Autodesk Inventor part; units mm, degrees
ref_plane "YZ Plane" through (0, 0, 0) normal (1, 0, 0) x (0, 1, 0)
ref_plane "XZ Plane" through (0, 0, 0) normal (0, 1, 0) x (-1, 0, 0)
ref_plane "XY Plane" through (0, 0, 0) normal (0, 0, 1) x (1, 0, 0)
sketch "Sketch1" plane through (0, 0, 0) normal (0, 0, 1) x (1, 0, 0)
  line L0 (6, 6) -> (200, 6)
  line L1 (200, 6) -> (200, 200)
  line L2 (200, 200) -> (42, 200)
  line L3 (6, 83) -> (6, 6)
  line L4 (6, 6) -> (56, 6)
  line L5 (200, 6) -> (150, 6)
  line L6 (200, 6) -> (200, 153)
  line L7 (150, 6) -> (142.5, 6)
  line L8 (200, 6) -> (200, 166)
  arc A0 (152.5, 174.3333) -> (147.5, 174.3333) centre (150, 174.3333) ccw
  line L9 (150, 6) -> (50, 6)
  arc A1 (47.8689, 14.6053) -> (52.8158, 14.5813) centre (50.3406, 14.23) ccw
  arc A2 (53.8259, 22.009) -> (52.8051, 13.8106) centre (86.918, 13.7258) ccw
  arc A3 (51.3944, 191.2047) -> (46.3962, 191.0801) centre (48.8946, 191.1682) ccw
  line L10 (53.8599, 22.4199) -> (51.3944, 191.2047)
  line L11 (48.8556, 22.7156) -> (46.3962, 191.0801)
  arc A4 (53.7373, 21.6465) -> (53.8589, 22.4929) centre (51.3599, 22.4199) ccw
  arc A5 (48.8556, 22.7156) -> (47.8689, 14.6053) centre (80.6169, 14.7362) ccw
  line L12 (52.8406, 14.23) -> (52.8088, 14.23)
  arc A6 (147.5, 14.23) -> (152.5, 14.23) centre (150, 14.23) ccw
  line L13 (147.5, 14.23) -> (147.5, 174.3333)
  line L14 (152.5, 14.23) -> (152.5, 174.3333)
  line L15 (42, 83) -> (6, 83)
  line L16 (42, 200) -> (39, 200)
  line L17 (39, 200) -> (39, 180)
  line L18 (39, 160) -> (39, 140)
  line L19 (39, 120) -> (39, 100)
  line L20 (39, 100) -> (42, 100)
  line L21 (39, 120) -> (42, 120)
  line L22 (39, 140) -> (42, 140)
  line L23 (39, 160) -> (42, 160)
  line L24 (39, 180) -> (42, 180)
  line L25 (39, 120) -> (39, 100)
  line L26 (39, 200) -> (39, 180)
  line L27 (39, 160) -> (39, 140)
  line L28 (42, 180) -> (42, 160)
  line L29 (42, 140) -> (42, 120)
  line L30 (42, 100) -> (42, 83)
  dimension "d1" = 194
extrude "Extrusion1" add sketch "Sketch1" along normal blind 3
sketch "Sketch2" plane through (0, 0, 3) normal (0, 0, 1) x (1, 0, 0)
  line L0 (200, 6) -> (200, 200)
  line L1 (200, 200) -> (39, 200)
  line L2 (42, 180) -> (42, 160)
  line L3 (42, 83) -> (6, 83)
  line L4 (6, 83) -> (6, 6)
  line L5 (6, 6) -> (200, 6)
  line L6 (147.5, 14.23) -> (147.5, 174.3333)
  arc A0 (152.5, 174.3333) -> (147.5, 174.3333) centre (150, 174.3333) ccw
  line L7 (152.5, 174.3333) -> (152.5, 14.23)
  arc A1 (147.5, 14.23) -> (152.5, 14.23) centre (150, 14.23) ccw
  arc A2 (51.3944, 191.2047) -> (46.3962, 191.0801) centre (48.8946, 191.1682) ccw
  line L8 (51.3944, 191.2047) -> (53.8589, 22.4929)
  arc A3 (53.7373, 21.6465) -> (53.8589, 22.4929) centre (51.3599, 22.4199) ccw
  arc A4 (53.7373, 21.6465) -> (52.8158, 14.5813) centre (86.918, 13.7258) ccw
  arc A5 (47.8689, 14.6053) -> (52.8158, 14.5813) centre (50.3406, 14.23) ccw
  arc A6 (48.8556, 22.7156) -> (47.8689, 14.6053) centre (80.6169, 14.7362) ccw
  line L9 (48.8556, 22.7156) -> (46.3962, 191.0801)
  line L10 (6, 6) -> (33, 6)
  line L11 (33, 6) -> (53, 6)
  line L12 (53, 6) -> (73, 6)
  line L13 (73, 6) -> (93, 6)
  line L14 (93, 6) -> (113, 6)
  line L15 (113, 6) -> (133, 6)
  line L16 (133, 6) -> (153, 6)
  line L17 (153, 6) -> (173, 6)
  line L18 (6, 6) -> (6, 9)
  line L19 (33, 6) -> (33, 3)
  line L20 (173, 6) -> (173, 3)
  line L21 (53, 6) -> (53, 3)
  line L22 (93, 6) -> (93, 3)
  line L23 (73, 6) -> (73, 3)
  line L24 (133, 6) -> (133, 3)
  line L25 (113, 6) -> (113, 3)
  line L26 (153, 6) -> (153, 3)
  line L27 (6, 6) -> (6, 3)
  line L28 (6, 3) -> (33, 3)
  line L29 (173, 3) -> (200, 3)
  line L30 (200, 3) -> (200, 6.6126)
  line L31 (73, 3) -> (53, 3)
  line L32 (153, 3) -> (133, 3)
  line L33 (113, 3) -> (93, 3)
  line L34 (39, 200) -> (39, 180)
  line L35 (39, 180) -> (42, 180)
  line L36 (42, 160) -> (39, 160)
  line L37 (39, 160) -> (39, 140)
  line L38 (39, 140) -> (42, 140)
  line L39 (42, 140) -> (42, 120)
  line L40 (42, 120) -> (39, 120)
  line L41 (39, 120) -> (39, 100)
  line L42 (39, 100) -> (42, 100)
  line L43 (42, 100) -> (42, 83)
  point P0 (120.702, 9)
  point P1 (49.056, 9)
extrude "Extrusion2" add sketch "Sketch2" against normal blind 3 contours L30 L29 L20 L5 | L26 L32 L24 L5 | L25 L33 L22 L5 | L23 L31 L21 L5 | L19 L28 L27 L5
sketch "Sketch3" plane through (0, 0, 3) normal (0, 0, 1) x (1, 0, 0)
  line L0 (153, 6) -> (173, 6)
  line L1 (113, 6) -> (133, 6)
  line L2 (200, 3) -> (200, 200)
  line L3 (200, 200) -> (39, 200)
  line L4 (42, 180) -> (42, 160)
  line L5 (42, 83) -> (6, 83)
  line L6 (6, 83) -> (6, 3)
  line L7 (73, 6) -> (93, 6)
  line L8 (33, 6) -> (53, 6)
  line L9 (147.5, 14.23) -> (147.5, 174.3333)
  arc A0 (152.5, 174.3333) -> (147.5, 174.3333) centre (150, 174.3333) ccw
  line L10 (152.5, 174.3333) -> (152.5, 14.23)
  arc A1 (147.5, 14.23) -> (152.5, 14.23) centre (150, 14.23) ccw
  arc A2 (51.3944, 191.2047) -> (46.3962, 191.0801) centre (48.8946, 191.1682) ccw
  line L11 (51.3944, 191.2047) -> (53.8589, 22.4929)
  arc A3 (53.7373, 21.6465) -> (53.8589, 22.4929) centre (51.3599, 22.4199) ccw
  arc A4 (53.7373, 21.6465) -> (52.8158, 14.5813) centre (86.918, 13.7258) ccw
  arc A5 (47.8689, 14.6053) -> (52.8158, 14.5813) centre (50.3406, 14.23) ccw
  arc A6 (48.8556, 22.7156) -> (47.8689, 14.6053) centre (80.6169, 14.7362) ccw
  line L12 (48.8556, 22.7156) -> (46.3962, 191.0801)
  line L13 (6, 83) -> (6, 80)
  line L14 (6, 83) -> (3, 83)
  line L15 (3, 6) -> (3, 14.5)
  line L16 (3, 83) -> (3, 74.5)
  line L17 (3, 54.5) -> (3, 34.5)
  line L18 (3, 74.5) -> (6, 74.5)
  line L19 (3, 54.5) -> (6, 54.5)
  line L20 (3, 34.5) -> (6, 34.5)
  line L21 (3, 14.5) -> (6, 14.5)
  line L22 (3, 14.5) -> (3, 6)
  line L23 (3, 83) -> (3, 74.5)
  line L24 (3, 54.5) -> (3, 34.5)
  line L25 (3, 6) -> (3, 3)
  line L26 (3, 3) -> (6, 3)
  line L27 (6, 3) -> (6, 6)
  line L28 (6, 3) -> (33, 3)
  line L29 (33, 3) -> (33, 6)
  line L30 (53, 6) -> (53, 3)
  line L31 (53, 3) -> (73, 3)
  line L32 (73, 3) -> (73, 6)
  line L33 (93, 6) -> (93, 3)
  line L34 (93, 3) -> (113, 3)
  line L35 (113, 3) -> (113, 6)
  line L36 (133, 6) -> (133, 3)
  line L37 (133, 3) -> (153, 3)
  line L38 (153, 3) -> (153, 6)
  line L39 (173, 6) -> (173, 3)
  line L40 (173, 3) -> (200, 3)
  line L41 (39, 200) -> (39, 180)
  line L42 (39, 180) -> (42, 180)
  line L43 (42, 160) -> (39, 160)
  line L44 (39, 160) -> (39, 140)
  line L45 (39, 140) -> (42, 140)
  line L46 (42, 140) -> (42, 120)
  line L47 (42, 120) -> (39, 120)
  line L48 (39, 120) -> (39, 100)
  line L49 (39, 100) -> (42, 100)
  line L50 (42, 100) -> (42, 83)
  point P0 (6, 3)
  dimension "d43" = 3
extrude "Extrusion3" add sketch "Sketch3" against normal blind 3 contours L26 L25 L15 L21 L6 | L6 L18 L16 L14 | L20 L17 L19 L6
sketch "Sketch4" plane through (0, 0, 3) normal (0, 0, 1) x (1, 0, 0)
  line L0 (153, 6) -> (173, 6)
  line L1 (113, 6) -> (133, 6)
  line L2 (200, 200) -> (39, 200)
  line L3 (42, 180) -> (42, 160)
  line L4 (42, 83) -> (3, 83)
  line L5 (3, 83) -> (3, 74.5)
  line L6 (3, 74.5) -> (6, 74.5)
  line L7 (6, 74.5) -> (6, 54.5)
  line L8 (6, 54.5) -> (3, 54.5)
  line L9 (3, 54.5) -> (3, 34.5)
  line L10 (3, 34.5) -> (6, 34.5)
  line L11 (73, 6) -> (93, 6)
  line L12 (33, 6) -> (53, 6)
  line L13 (147.5, 14.23) -> (147.5, 174.3333)
  arc A0 (152.5, 174.3333) -> (147.5, 174.3333) centre (150, 174.3333) ccw
  line L14 (152.5, 174.3333) -> (152.5, 14.23)
  arc A1 (147.5, 14.23) -> (152.5, 14.23) centre (150, 14.23) ccw
  arc A2 (51.3944, 191.2047) -> (46.3962, 191.0801) centre (48.8946, 191.1682) ccw
  line L15 (51.3944, 191.2047) -> (53.8589, 22.4929)
  arc A3 (53.7373, 21.6465) -> (53.8589, 22.4929) centre (51.3599, 22.4199) ccw
  arc A4 (53.7373, 21.6465) -> (52.8158, 14.5813) centre (86.918, 13.7258) ccw
  arc A5 (47.8689, 14.6053) -> (52.8158, 14.5813) centre (50.3406, 14.23) ccw
  arc A6 (48.8556, 22.7156) -> (47.8689, 14.6053) centre (80.6169, 14.7362) ccw
  line L16 (48.8556, 22.7156) -> (46.3962, 191.0801)
  line L17 (200, 200) -> (203, 200)
  line L18 (200, 6) -> (200, 33)
  line L19 (200, 33) -> (200, 53)
  line L20 (200, 53) -> (200, 73)
  line L21 (200, 73) -> (200, 93)
  line L22 (200, 93) -> (200, 113)
  line L23 (200, 113) -> (200, 133)
  line L24 (200, 133) -> (200, 153)
  line L25 (200, 153) -> (200, 173)
  line L26 (200, 173) -> (200, 200)
  line L27 (200, 173) -> (203, 173)
  line L28 (200, 153) -> (203, 153)
  line L29 (200, 133) -> (203, 133)
  line L30 (200, 113) -> (203, 113)
  line L31 (200, 93) -> (203, 93)
  line L32 (200, 73) -> (203, 73)
  line L33 (200, 53) -> (203, 53)
  line L34 (200, 33) -> (203, 33)
  line L35 (203, 200) -> (203, 173)
  line L36 (203, 153) -> (203, 133)
  line L37 (203, 113) -> (203, 93)
  line L38 (203, 73) -> (203, 53)
  line L39 (203, 33) -> (203, 6)
  line L40 (200, 3) -> (200, 200)
  line L41 (6, 34.5) -> (6, 14.5)
  line L42 (3, 3) -> (33, 3)
  line L43 (33, 3) -> (33, 6)
  line L44 (53, 6) -> (53, 3)
  line L45 (53, 3) -> (73, 3)
  line L46 (73, 3) -> (73, 6)
  line L47 (93, 6) -> (93, 3)
  line L48 (93, 3) -> (113, 3)
  line L49 (113, 3) -> (113, 6)
  line L50 (133, 6) -> (133, 3)
  line L51 (133, 3) -> (153, 3)
  line L52 (153, 3) -> (153, 6)
  line L53 (173, 6) -> (173, 3)
  line L54 (173, 3) -> (200, 3)
  line L55 (6, 14.5) -> (3, 14.5)
  line L56 (3, 14.5) -> (3, 3)
  line L57 (200, 3) -> (203, 3)
  line L58 (203, 3) -> (203, 6)
  line L59 (39, 200) -> (39, 180)
  line L60 (39, 180) -> (42, 180)
  line L61 (42, 160) -> (39, 160)
  line L62 (39, 160) -> (39, 140)
  line L63 (39, 140) -> (42, 140)
  line L64 (42, 140) -> (42, 120)
  line L65 (42, 120) -> (39, 120)
  line L66 (39, 120) -> (39, 100)
  line L67 (39, 100) -> (42, 100)
  line L68 (42, 100) -> (42, 83)
extrude "Extrusion4" add sketch "Sketch4" against normal blind 3 contours L40 L18 L34 L39 L58 L57 | L20 L32 L38 L33 | L22 L30 L37 L31 | L24 L28 L36 L29 | L26 L17 L35 L27
sketch "Sketch7" plane through (0, 0, 3) normal (0, 0, 1) x (1, 0, 0)
  line L0 (6, 60) -> (18, 60)
  line L1 (18, 60) -> (18, 50)
  line L2 (18, 50) -> (6, 50)
  line L3 (6, 50) -> (6, 60)
  line L4 (6, 60) -> (18, 50) construction
  line L5 (18, 60) -> (6, 50) construction
  line L6 (12, 55) -> (7.5, 55)
  line L7 (7.5, 55) -> (16.5, 55)
  circle A0 centre (7.5, 55) radius 0.625
  circle A1 centre (16.5, 55) radius 0.625
  line L8 (6.875, 55) -> (12, 55)
  circle A2 centre (12, 55) radius 2.25
  dimension "d74" = 1.25
  dimension "d70" = 12
  dimension "d71" = 10
  dimension "d72" = 4.5
  dimension "d73" = 9
  dimension "d75" = 1.25
  dimension "d78" = 4.5
extrude "Extrusion5" cut sketch "Sketch7" against normal blind 3 contours A2 L7 L6 | L6 L7 A2
sketch "Sketch8" plane through (0, 0, 3) normal (0, 0, 1) x (1, 0, 0)
  circle A0 centre (12, 55) radius 2.25
  line L0 (12, 55) -> (12, 96)
  circle A1 centre (12, 55) radius 2.25
  line L1 (200, 33) -> (200, 53)
  line L2 (200, 53) -> (203, 53)
  line L3 (203, 53) -> (203, 73)
  line L4 (203, 73) -> (200, 73)
  line L5 (200, 73) -> (200, 93)
  line L6 (200, 93) -> (203, 93)
  line L7 (203, 93) -> (203, 113)
  line L8 (203, 113) -> (200, 113)
  line L9 (200, 113) -> (200, 133)
  line L10 (200, 133) -> (203, 133)
  line L11 (203, 133) -> (203, 153)
  line L12 (203, 153) -> (200, 153)
  line L13 (200, 153) -> (200, 173)
  line L14 (200, 173) -> (203, 173)
  line L15 (203, 173) -> (203, 200)
  line L16 (203, 200) -> (39, 200)
  line L17 (42, 180) -> (42, 160)
  line L18 (42, 83) -> (3, 83)
  line L19 (3, 83) -> (3, 74.5)
  line L20 (3, 74.5) -> (6, 74.5)
  line L21 (6, 74.5) -> (6, 54.5)
  line L22 (6, 54.5) -> (3, 54.5)
  line L23 (3, 54.5) -> (3, 34.5)
  line L24 (3, 34.5) -> (6, 34.5)
  line L25 (6, 34.5) -> (6, 14.5)
  line L26 (6, 14.5) -> (3, 14.5)
  line L27 (3, 14.5) -> (3, 3)
  line L28 (3, 3) -> (33, 3)
  line L29 (33, 3) -> (33, 6)
  line L30 (33, 6) -> (53, 6)
  line L31 (53, 6) -> (53, 3)
  line L32 (53, 3) -> (73, 3)
  line L33 (73, 3) -> (73, 6)
  line L34 (73, 6) -> (93, 6)
  line L35 (93, 6) -> (93, 3)
  line L36 (93, 3) -> (113, 3)
  line L37 (113, 3) -> (113, 6)
  line L38 (113, 6) -> (133, 6)
  line L39 (133, 6) -> (133, 3)
  line L40 (133, 3) -> (153, 3)
  line L41 (153, 3) -> (153, 6)
  line L42 (153, 6) -> (173, 6)
  line L43 (173, 6) -> (173, 3)
  line L44 (173, 3) -> (203, 3)
  line L45 (203, 3) -> (203, 33)
  line L46 (203, 33) -> (200, 33)
  line L47 (147.5, 14.23) -> (147.5, 174.3333)
  arc A2 (152.5, 174.3333) -> (147.5, 174.3333) centre (150, 174.3333) ccw
  line L48 (152.5, 174.3333) -> (152.5, 14.23)
  arc A3 (147.5, 14.23) -> (152.5, 14.23) centre (150, 14.23) ccw
  arc A4 (51.3944, 191.2047) -> (46.3962, 191.0801) centre (48.8946, 191.1682) ccw
  line L49 (51.3944, 191.2047) -> (53.8589, 22.4929)
  arc A5 (53.7373, 21.6465) -> (53.8589, 22.4929) centre (51.3599, 22.4199) ccw
  arc A6 (53.7373, 21.6465) -> (52.8158, 14.5813) centre (86.918, 13.7258) ccw
  arc A7 (47.8689, 14.6053) -> (52.8158, 14.5813) centre (50.3406, 14.23) ccw
  arc A8 (48.8556, 22.7156) -> (47.8689, 14.6053) centre (80.6169, 14.7362) ccw
  line L50 (48.8556, 22.7156) -> (46.3962, 191.0801)
  line L51 (42, 83) -> (3, 83)
  line L52 (12, 55) -> (42, 83)
  arc A9 (42, 83) -> (12, 96) centre (12.05, 55) ccw
  line L53 (3, 83) -> (6, 83)
  line L54 (6, 83) -> (6, 96)
  line L55 (6, 96) -> (12, 96)
  line L56 (6, 83) -> (42, 83)
  line L57 (39, 200) -> (39, 180)
  line L58 (39, 180) -> (42, 180)
  line L59 (42, 160) -> (39, 160)
  line L60 (39, 160) -> (39, 140)
  line L61 (39, 140) -> (42, 140)
  line L62 (42, 140) -> (42, 120)
  line L63 (42, 120) -> (39, 120)
  line L64 (39, 120) -> (39, 100)
  line L65 (39, 100) -> (42, 100)
  line L66 (42, 100) -> (42, 83)
  dimension "d79" = 41
  dimension "d80" = 41
  dimension "d81" = 3
  dimension "d82" = 13
extrude "Extrusion6" add sketch "Sketch8" against normal blind 3 contours L18 L0 A9 | L18 L54 L55 L0
properties part number "inside walls"
Part model, mm, in its own coordinate system. Round coordinates to 2 decimals unless told otherwise and drop trailing zeros. Loops run counter-clockwise (first coordinate to the right, second up) from the corner with the lowest first, then second, coordinate; pieces in that order, holes last.
Item 1: Cut at A-A, the plane z = 2.2. State how many separate pieces and enclosed holes the cut face has, then the cut area to 3 significant figures.
Item 2: Cut at B-B, the plane x = 166. Give the cut face in (y, z), then the cut area to 3 significant figures.
Item 3: Drop flat-ended pins along their axis: P1, Ø1.5, axis at x = 46, z = 1.5, coming from the -Y side; P2, Ø4, axis at x = 12, y = 55, coming from the +Z side; P3, Ø1.5, axis at y = 96, z = 1.5, coming from the -X side; P4, Ø0.9, axis at y = 131, z = 1, coming from the -X side. Give the stop position or say it passes through.
Item 4: Cut at C-C, the plane x = 18. Give the cut face in (y, z), then the cut area to 3 significant figures.
Item 5: Mould opens along Y. For faces 1 (the face through (11.71, 57.23, 1.52)), 2 (the face through (102, 103, 3)) say: +Y half, -Y half, draft (parallel to the pull), parting line (faces both ways), or undercut.
Item 6: Drill centre lines: line 1 (X direction, y = 55, z = 0.7); line 2 (X direction, y = 19.5, z = 1.7); line 3 (X direction, y = 84.5, z = 2.8). Where is each one in solid material? Low to high.
A:
1. separate pieces: 1
1. enclosed holes: 3
1. area: 33,000 mm2
2. outline: (6, 0) - (200, 0) - (200, 3) - (6, 3) - close
2. area: 582 mm2
3. P1: stops at y = 6
3. P2: passes through
3. P3: stops at x = 6
3. P4: stops at x = 42
4. outline: (3, 0) - (95.57, 0) - (95.57, 3) - (3, 3) - close
4. area: 278 mm2
5. face 1: undercut
5. face 2: draft
6. line 1: x = 6 to 9.75, 14.25 to 48.38, 53.38 to 147.5, 152.5 to 203
6. line 2: x = 6 to 48.22, 53.3 to 147.5, 152.5 to 203
6. line 3: x = 6 to 40.52, 42 to 47.95, 52.95 to 147.5, 152.5 to 200
